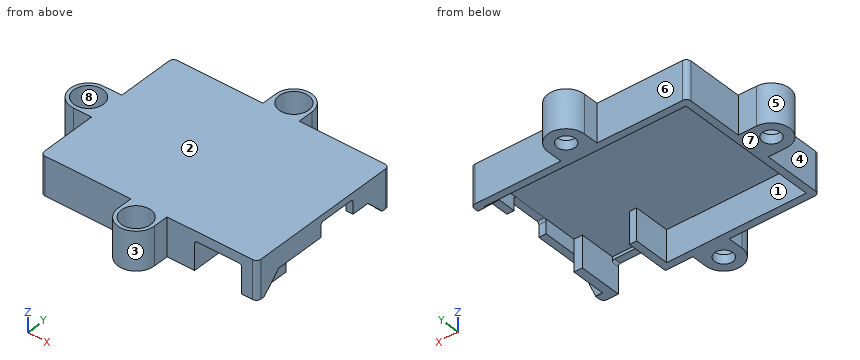
from build123d import *

# Parameters (mm, degrees)
SKETCH1_W           = 47.85
SKETCH1_H           = 35.2
SKETCH1_W_2         = 44.65
SKETCH1_H_2         = 32
BOSS_EXTRUDE1_DEPTH = 6.99
SKETCH2_W           = 47.85
SKETCH2_H           = 35.2
BOSS_EXTRUDE2_DEPTH = 1.5
CUT_EXTRUDE1_REACH  = 53.686
SKETCH4_W           = 3.5
SKETCH4_H           = 8.5
CUT_EXTRUDE2_DEPTH  = 1.6
CUT_EXTRUDE3_REACH  = 45.4
SKETCH6_W           = 10.4
SKETCH6_H           = 6.6
FILLET1_R           = 1
FILLET2_R           = 0.5
SKETCH7_R           = 2
BOSS_EXTRUDE3_DEPTH = 8.49
SKETCH8_R           = 3.25
CUT_EXTRUDE4_DEPTH  = 6.49
BOSS_EXTRUDE4_REACH = 43.428
SKETCH9_W           = 1.6
SKETCH9_H           = 8
SKETCH9_W_2         = 1.845


with BuildPart() as part:
    # Sketch1 → Boss-Extrude1 (new body)
    with BuildSketch(Plane.XY):
        Rectangle(SKETCH1_W, SKETCH1_H)
        Rectangle(SKETCH1_W_2, SKETCH1_H_2, mode=Mode.SUBTRACT)
    extrude(amount=BOSS_EXTRUDE1_DEPTH)

    # Sketch2 → Boss-Extrude2 (add)
    with BuildSketch(Plane.XY.offset(6.99)):
        Rectangle(SKETCH2_W, SKETCH2_H)
    extrude(amount=BOSS_EXTRUDE2_DEPTH)

    # Sketch3 → Cut-Extrude1 (cut, up to next)
    with BuildSketch(Plane(origin=(23.925, 0, 0), x_dir=(0, 0, -1), z_dir=(1, 0, 0)), mode=Mode.PRIVATE) as cut_extrude1_sk1:
        Polygon((-0.070710678, 15.670710678), (0, 15.670710678), (0, -15.670710678), (-0.070710678, -15.670710678), (-3.85, -11.891421356), (-3.85, 11.891421356), align=None)
    cut_extrude1_tool1 = extrude(cut_extrude1_sk1.sketch, amount=-CUT_EXTRUDE1_REACH, mode=Mode.PRIVATE) & part.part
    add(cut_extrude1_tool1.solids().sort_by_distance((23.925, 0, 1.835684))[0], mode=Mode.SUBTRACT)

    # Sketch4 → Cut-Extrude2 (cut)
    with BuildSketch(Plane(origin=(23.925, 0, 0), x_dir=(0, 0, -1), z_dir=(1, 0, 0))):
        with Locations((-5.25, 3.670508357)):
            Rectangle(SKETCH4_W, SKETCH4_H)
    extrude(amount=-CUT_EXTRUDE2_DEPTH, mode=Mode.SUBTRACT)

    # Sketch6 → Cut-Extrude3 (cut, up to next)
    with BuildSketch(Plane.XZ.offset(17.6), mode=Mode.PRIVATE) as cut_extrude3_sk1:
        with Locations((15.28, 3.02)):
            Rectangle(SKETCH6_W, SKETCH6_H)
    cut_extrude3_tool1 = extrude(cut_extrude3_sk1.sketch, amount=-CUT_EXTRUDE3_REACH, mode=Mode.PRIVATE) & part.part
    add(cut_extrude3_tool1.solids().sort_by_distance((15.28, -17.6, 3.02))[0], mode=Mode.SUBTRACT)

    # Fillet1
    fillet1_edges = [part.edges().sort_by_distance(p)[0] for p in [
        (-23.925, 17.6, 4.245),
        (23.925, 17.6, 4.245),
        (23.925, -17.6, 4.245),
        (-23.925, -17.6, 4.245),
    ]]
    fillet(fillet1_edges, radius=FILLET1_R)

    # Fillet2
    # the kernel refuses this fillet: 0.5 mm, written as the material it adds along each edge
    with BuildSketch(Plane(origin=(20.48, -17.6, 6.32), x_dir=(-1, 0, 0), z_dir=(0, 1, 0)), Plane(origin=(10.08, -17.6, 6.32), x_dir=(0, 0, -1), z_dir=(0, 1, 0)), Plane(origin=(23.925, 7.920508357, 7), x_dir=(0, -1, 0), z_dir=(-1, 0, 0)), Plane(origin=(23.925, -0.579491643, 7), x_dir=(0, 0, -1), z_dir=(-1, 0, 0))) as fillet2_piece_1:
        with BuildLine():
            CenterArc((FILLET2_R, -FILLET2_R), FILLET2_R, 90, 90)
            Line((0, -FILLET2_R), (0, 0))
            Line((0, 0), (FILLET2_R, 0))
        make_face()
    extrude(amount=1.6)

    # Sketch7 → Boss-Extrude3 (add)
    # profile 1 of 3: a face of its own
    with BuildSketch(Plane.XY.offset(8.49)):
        with BuildLine():
            Line((4, -17.6), (4, -21))
            ThreePointArc((4, -21), (0, -25), (-4, -21))
            Line((-4, -21), (-4, -17.6))
            Line((-4, -17.6), (4, -17.6))
        make_face()
        with Locations((0, -21)):
            Circle(SKETCH7_R, mode=Mode.SUBTRACT)
    # profile 2 of 3: a face of its own
    with BuildSketch(Plane.XY.offset(8.49)):
        with BuildLine():
            Line((-4, 17.6), (-4, 21))
            ThreePointArc((-4, 21), (0, 25), (4, 21))
            Line((4, 21), (4, 17.6))
            Line((4, 17.6), (-4, 17.6))
        make_face()
        with Locations((0, 21)):
            Circle(SKETCH7_R, mode=Mode.SUBTRACT)
    # profile 3 of 3: a face of its own
    with BuildSketch(Plane.XY.offset(8.49)):
        with BuildLine():
            Line((-23.925, -4), (-27.925, -4))
            ThreePointArc((-27.925, -4), (-31.925, 0), (-27.925, 4))
            Line((-27.925, 4), (-23.925, 4))
            Line((-23.925, 4), (-23.925, -4))
        make_face()
        with Locations((-27.925, 0)):
            Circle(SKETCH7_R, mode=Mode.SUBTRACT)
    extrude(amount=-BOSS_EXTRUDE3_DEPTH)

    # Sketch8 → Cut-Extrude4 (cut)
    with BuildSketch(Plane.XY.offset(8.49)):
        with Locations((0, 21)):
            Circle(SKETCH8_R)
        with Locations((0, -21)):
            Circle(SKETCH8_R)
        with Locations((-27.925, 0)):
            Circle(SKETCH8_R)
    extrude(amount=-CUT_EXTRUDE4_DEPTH, mode=Mode.SUBTRACT)

    # Boss-Extrude4: up to this face of the body (flat: up to its plane)
    boss_extrude4_end = Plane(part.part.faces().sort_by_distance((0, 0, 6.99))[0])
    # Sketch9 → Boss-Extrude4 (add, up to the picked face)
    with BuildSketch(Plane(origin=(0, 0, 0), x_dir=(-1, 0, 0), z_dir=(0, 0, -1)), mode=Mode.PRIVATE) as boss_extrude4_sk1:
        with Locations((-9.28, -12)):
            Rectangle(SKETCH9_W, SKETCH9_H)
    boss_extrude4_tool1 = split(extrude(boss_extrude4_sk1.sketch, amount=-BOSS_EXTRUDE4_REACH, mode=Mode.PRIVATE), bisect_by=boss_extrude4_end, keep=Keep.BOTH, mode=Mode.PRIVATE)
    # Sketch9 → Boss-Extrude4 (add, up to the picked face)
    with BuildSketch(Plane(origin=(0, 0, 0), x_dir=(-1, 0, 0), z_dir=(0, 0, -1)), mode=Mode.PRIVATE) as boss_extrude4_sk2:
        with Locations((-21.4025, -12)):
            Rectangle(SKETCH9_W_2, SKETCH9_H)
    boss_extrude4_tool2 = split(extrude(boss_extrude4_sk2.sketch, amount=-BOSS_EXTRUDE4_REACH, mode=Mode.PRIVATE), bisect_by=boss_extrude4_end, keep=Keep.BOTH, mode=Mode.PRIVATE)
    add(boss_extrude4_tool1.solids().sort_by(Axis((9.28, -12, 0), (0, 0, 1)))[0])
    add(boss_extrude4_tool2.solids().sort_by(Axis((21.4025, -12, 0), (0, 0, 1)))[0])


solid = part.part
Model file for the job. Use its own axes, mm. Face numbers are marked on the shaded views. A direction names the side the tool comes from. Coordinates: 2 decimals unless noted, no trailing zeros. Write each loop counter-clockwise with the first axis right and the second up, starting at its lowest first coordinate (ties: lowest second). Pieces come first, ordered by that corner, then holes. Notation, with made-up numbers: (80.25, 80.25) -> (85.25, 80.25) arc R18 ccw to (85.25, 95.25) -> close; hole circle Ø9 at (55, 77). An arc over 180 degrees is marked (long way). One line per item, written item: value. Start each with the question number.
1) Slice it at C-C on y = 6.5. Write the cut outline in (x, z) (3 decimals).
2) Slice it at B-B on x = 0. Write the cut outline in (y, z), then the cut area to 3 significant figures.
3) Probe probe 1 along Y at (x, z) = (0, 7.25); probe 2 along Y at (x, z) = (0, 4.75); probe 3 along X at (y, z) = (-15.5, 3.5) (3 decimals). List the from-to ranges inside material, lowest first.
4) Which spindle directions (+Z, -Z, +X, -X, +Y, -Y) get a long thin tool onto all of the face, cutting with end or side? Do the marked faces 4, 5, 6, 7 and 8. Say none if no direction does.
5) Flat gauge pins, fed straight in: pin 1 Ø2 at (x, z) = (-5.5, 3) entering from -Y; pin 2 Ø10 at (x, y) = (4.5, 14.5) entering from -Z; pin 3 Ø2.5 at (y, z) = (-19, 2.5) entering from -X; pin 4 Ø8 at (x, y) = (5.5, -4.5) entering from -Z. Where does each tip first touch, or does it go through?
6) Pull direction X, two halves, no side cores. Call the marked faces 1, 2 and 3: +X half, -X half, draft (parallel to the pull), parting line (faces both ways), or undercut.
7) Slice it at A-A on x = 12. Write the cut outline in (y, z), then the cut area to 3 significant figures.
8) Slice it at D-D on z = 1. Count the separate pieces of the cut face and the enclosed holes in it, then the cut area to 3 significant figures.
Answers follow:
1. outline: (-23.925, 0) -> (-22.325, 0) -> (-22.325, 6.99) -> (22.325, 6.99) -> (22.325, 7) -> (23.925, 7) -> (23.925, 8.49) -> (-23.925, 8.49) -> close
2. outline: (-25, 0) -> (-23, 0) -> (-23, 2) -> (-24.25, 2) -> (-24.25, 8.49) -> (-25, 8.49) -> close; (-19, 0) -> (-16, 0) -> (-16, 6.99) -> (16, 6.99) -> (16, 0) -> (19, 0) -> (19, 2) -> (17.75, 2) -> (17.75, 8.49) -> (-17.75, 8.49) -> (-17.75, 2) -> (-19, 2) -> close; (23, 0) -> (25, 0) -> (25, 8.49) -> (24.25, 8.49) -> (24.25, 2) -> (23, 2) -> close
2. area: 100 mm2
3. probe 1: -25 to -24.25, -17.75 to 17.75, 24.25 to 25
3. probe 2: -25 to -24.25, -17.75 to -16, 16 to 17.75, 24.25 to 25
3. probe 3: -23.925 to -22.325, 8.48 to 10.08, 20.48 to 23.925
4. face 4: +Z, -Z, -X, -Y
4. face 5: +Z, -Z, -X
4. face 6: +Z, -Z, -X, +Y
4. face 7: -Z, +X, -X, +Y, -Y
4. face 8: +Z
5. pin 1: y = -17.6
5. pin 2: z = 0
5. pin 3: x = -4
5. pin 4: z = 6.99
6. face 1: undercut
6. face 2: draft
6. face 3: parting line
7. outline: (-17.6, 6.32) -> (-16, 6.32) -> (-16, 6.99) -> (16, 6.99) -> (16, 0) -> (17.6, 0) -> (17.6, 8.49) -> (-17.6, 8.49) -> close
7. area: 65.1 mm2
8. separate pieces: 2
8. enclosed holes: 3
8. area: 343 mm2
